Autodesk Inventor part; units mm, degrees
ref_plane "YZ Plane" through (0, 0, 0) normal (1, 0, 0) x (0, 1, 0)
ref_plane "XZ Plane" through (0, 0, 0) normal (0, 1, 0) x (-1, 0, 0)
ref_plane "XY Plane" through (0, 0, 0) normal (0, 0, 1) x (1, 0, 0)
sketch "スケッチ1" plane through (0, 0, 0) normal (0, 1, 0) x (-1, 0, 0)
  line L0 (0, 0) -> (25, 0)
  line L1 (25, 0) -> (25, -25)
  line L2 (25, -25) -> (0, -25)
  line L3 (0, -25) -> (0, 0)
  dimension "d0" = 25
  dimension "d1" = 25
extrude "押し出し1" add sketch "スケッチ1" along normal blind 5
sketch "スケッチ2" plane through (0, 5, 0) normal (0, 1, 0) x (1, 0, 0)
  line L0 (-25, 0) -> (0, 0)
  line L1 (0, 0) -> (0, 25)
  line L2 (0, 25) -> (-25, 25)
  line L3 (-25, 25) -> (-25, 0)
  point P0 (-2.5, 2.5)
  point P1 (-2.5, 2.5)
  point P2 (-2.5, 22.5)
  point P3 (-22.4998, 22.5838)
  point P4 (-22.4998, 2.5838)
  dimension "d4" = 2.5
  dimension "d5" = 2.5
  dimension "d6" = 20
  dimension "d7" = 20
  dimension "d8" = 20
  dimension "d9" = 20
  dimension "d10" = 2.5
  dimension "d12" = 2.5002
hole "穴1" at (-2.5, 5, -2.5) at (-2.5, 5, -22.5) at (-22.4998, 5, -22.5838) at (-22.4998, 5, -2.5838) direction (0, -1, 0) diameter 3.6 end through all
properties part number "Plate5mmforPrint2"
CAD build for the part. Positions are in the model's coordinates, mm. Give positions to 0.01 mm unless a question says otherwise; leave off trailing zeros. Order: outer loops, then holes, each group sorted by start corner. A loop starts at its lowest first (then second) coordinate and runs counter-clockwise, first axis right, second up. Notation, with made-up numbers: (21.25, 46) -> (52.25, 46) arc R16 cw to (52.25, 62) -> close; hole circle Ø4 at (-17, 69.5). An arc over 180 degrees is marked (long way). Return JSON: item names as keys, results as strings.
Q1. Saw through at C-C (y = 3.7). Write the cut outline in (x, z), then the cut area to 3 significant figures.
Working result:
{"outline": "(-25, -25) -> (0, -25) -> (0, 0) -> (-25, 0) -> close; hole circle Ø3.6 at (-22.5, -22.58); hole circle Ø3.6 at (-22.5, -2.58); hole circle Ø3.6 at (-2.5, -22.5); hole circle Ø3.6 at (-2.5, -2.5)", "area": "584 mm²"}
Q2. Saw through at A-A (x = -2.5). Write the cut outline in (y, z), then the cut area to 3 significant figures.
Working result:
{"outline": "(0, -25) -> (5, -25) -> (5, -24.3) -> (0, -24.3) -> close; (0, -20.7) -> (5, -20.7) -> (5, -4.3) -> (0, -4.3) -> close; (0, -0.7) -> (5, -0.7) -> (5, 0) -> (0, 0) -> close", "area": "89.0 mm²"}
Q3. Drill centre lines: line 1 (Z direction, x = -2.5, y = 1.6); line 2 (X direction, y = 3.65, z = -21.5). Where is each one in solid material? Low to high.
Working result:
{"line 1": "-25 to -24.3, -20.7 to -4.3, -0.7 to 0", "line 2": "-25 to -23.94, -21.06 to -4, -1 to 0"}
Q4. Flat gauge pin, fed straight in: pin 1 (2 mm diameter, centred on x = -2.5, z = -22.5, fed in from +Y). Where does the tip first touch, or does it go through?
Working result:
{"pin 1": "through"}
Q5. Mould opens along X. For faces 1 (the face through (-12, 0, -12)), 2 (the face through (-25, 2, -12)), 3 (the face through (-3.041, 2.465, -20.783)) say: pulls with the +X half, pulls with the -X half, needs draft (parallel to the pull), parting line crosses it, or undercut.
Working result:
{"face 1": "needs draft", "face 2": "pulls with the -X half", "face 3": "undercut"}
Q6. Saw through at B-B (z = -2.5). Write the cut outline in (x, y).
Working result:
{"outline": "(-25, 0) -> (-24.3, 0) -> (-24.3, 5) -> (-25, 5) -> close; (-20.7, 0) -> (-4.3, 0) -> (-4.3, 5) -> (-20.7, 5) -> close; (-0.7, 0) -> (0, 0) -> (0, 5) -> (-0.7, 5) -> close"}
